Geometry: final body of the model. Coordinates: model frame, mm. A direction names the side the tool comes from. Round coordinates to 2 decimals unless told otherwise and drop trailing zeros. Order: outer loops, then holes, each group sorted by start corner. A loop starts at its lowest first (then second) coordinate and runs counter-clockwise, first axis right, second up. Notation, with made-up numbers: (9.25, 21.5) -> (45.25, 21.5) arc R14 cw to (45.25, 48.5) -> close; hole circle Ø3 at (-12.5, -37.5). An arc over 180 degrees is marked (long way). Put each result on its own line as item: value.
```python
from build123d import *

# Parameters (mm, degrees)
ESQUISSE1_R             = 1.5
BOSS_EXTRU_1_DEPTH      = 1.5
ESQUISSE2_R             = 0.75
BOSS_EXTRU_2_DEPTH      = 25.5
ESQUISSE3_W             = 0.5
ESQUISSE3_H             = 0.5
ENL_V_MAT_EXTRU_1_DEPTH = 1
CONG_1_R                = 0.5


with BuildPart() as part:
    # Esquisse1 → Boss.-Extru.1 (new body)
    with BuildSketch(Plane.XZ.offset(1.5)):
        with Locations(Location((-17.069271079, 10.656506254, 0), (0, 0, 270))):
            Circle(ESQUISSE1_R)
    extrude(amount=-BOSS_EXTRU_1_DEPTH)

    # Esquisse2 → Boss.-Extru.2 (add)
    with BuildSketch(Plane(origin=(0, 0, 0), x_dir=(1, 0, 0), z_dir=(0, 1, 0))):
        with Locations(Location((-17.069271079, -10.656506254, 0), (0, 0, 90))):
            Circle(ESQUISSE2_R)
    extrude(amount=BOSS_EXTRU_2_DEPTH)

    # Esquisse3 → Enlèv. mat.-Extru.1 (cut)
    with BuildSketch(Plane.XZ.offset(1.5)):
        with BuildLine():
            Line((-16.819271079, 9.177486308), (-16.819271079, 10.406506254))
            Line((-16.819271079, 10.406506254), (-17.319271079, 10.406506254))
            Line((-17.319271079, 10.406506254), (-17.319271079, 9.177486308))
            ThreePointArc((-17.319271079, 9.177486308), (-17.069271079, 9.156506254), (-16.819271079, 9.177486308))
        make_face()
        with BuildLine():
            Line((-16.819271079, 10.906506254), (-16.819271079, 12.1355262))
            ThreePointArc((-16.819271079, 12.1355262), (-17.069271079, 12.156506254), (-17.319271079, 12.1355262))
            Line((-17.319271079, 12.1355262), (-17.319271079, 10.906506254))
            Line((-17.319271079, 10.906506254), (-16.819271079, 10.906506254))
        make_face()
        with BuildLine():
            Line((-15.590251133, 10.906506254), (-16.819271079, 10.906506254))
            Line((-16.819271079, 10.906506254), (-16.819271079, 10.406506254))
            Line((-16.819271079, 10.406506254), (-15.590251133, 10.406506254))
            ThreePointArc((-15.590251133, 10.406506254), (-15.574525295, 10.531066863), (-15.569271079, 10.656506254))
            ThreePointArc((-15.569271079, 10.656506254), (-15.574525295, 10.781945644), (-15.590251133, 10.906506254))
        make_face()
        with BuildLine():
            Line((-17.319271079, 10.406506254), (-17.319271079, 10.906506254))
            Line((-17.319271079, 10.906506254), (-18.548291025, 10.906506254))
            ThreePointArc((-18.548291025, 10.906506254), (-18.569271079, 10.656506254), (-18.548291025, 10.406506254))
            Line((-18.548291025, 10.406506254), (-17.319271079, 10.406506254))
        make_face()
        with Locations((-17.069271079, 10.656506254)):
            Rectangle(ESQUISSE3_W, ESQUISSE3_H)
    extrude(amount=-ENL_V_MAT_EXTRU_1_DEPTH, mode=Mode.SUBTRACT)

    # Congé1
    cong_1_edges = [part.edges().sort_by_distance(p)[0] for p in [
        (-16.008610907, -1.5, 11.717166426),
        (-18.129931251, -1.5, 11.717166426),
        (-18.129931251, -1.5, 9.595846082),
        (-16.008610907, -1.5, 9.595846082),
    ]]
    fillet(cong_1_edges, radius=CONG_1_R)


solid = part.part
```
1. Set-up query: faces 1 (the face through (-17, 25.5, 11)), 2 (the face through (-18, -1, 10.407)), 3 (the face through (-16.404, 12.572, 10.31)), 4 (the face through (-17.319, -1, 10)). Return all of +Z, -Z, +X, -X, +Y, -Y with unobstructed straight access to the full face (end or side cutting, diameter ignored); none if empty.
Ans:
face 1: +Z, -Z, +X, -X, +Y
face 2: +X, -X, -Y
face 3: +Y
face 4: +Z, -Z, -Y
2. Contact query for flat-ended pins moving along their axis: P1, Ø1, axis at y = 7.5, z = 11.5, coming from the +X side; P2, Ø0.5, axis at x = -18, y = -1, coming from the -Z side; P3, Ø0.5, axis at x = -16.5, y = -1, coming from the -Z side; P4, Ø1.5, axis at x = -17, z = 11, coming from the -Y side. Output: stop coordinate, or through.
Ans:
P1: x = -16.4
P2: z = 9.32
P3: z = 9.19
P4: y = -1.5
3. Material intervals for probe 1 along Y at (x, z) = (-16.95, 11.55); probe 2 along Y at (x, z) = (-17.9, 11); probe 3 along Z at (x, y) = (-17, 13.5), sorted ascending.
Ans:
probe 1: -0.5 to 0
probe 2: -1.5 to 0
probe 3: 9.91 to 11.4
4. Cut plane A-A on y = 20.75. Return loops of the section in (x, z).
Ans:
outline: circle Ø1.5 at (-17.07, 10.66)
5. Draft query along Z for faces 5 (the face through (-16, -1, 10.907)), 6 (the face through (-17.319, -1, 11.5)), 7 (the face through (-17.64, -0.51, 9.27)), 8 (the face through (-16, -1, 10.407)). Return one class per face: +Z half, -Z half, draft (parallel to the pull), parting line (faces both ways), or undercut.
Ans:
face 5: undercut
face 6: draft
face 7: parting line
face 8: undercut
